Verification items for the finished model (mm, model axes). Give positions to 0.01 mm unless a question says otherwise; leave off trailing zeros. Write each loop counter-clockwise with the first axis right and the second up, starting at its lowest first coordinate (ties: lowest second). Pieces come first, ordered by that corner, then holes. Notation, with made-up numbers: (49, 38.5) -> (64, 38.5) arc R20 ccw to (64, 60.5) -> close; hole circle Ø1 at (-15.5, 3). An arc over 180 degrees is marked (long way). Use CSV: the item, a comma, the result in double quotes. Start each with the question number.
```python
from build123d import *

# Parameters (mm, degrees)
SKETCH_1_R              = 50
EXTRUDE_1_DEPTH         = 3.302
SKETCH_2_R              = 4.064
CUT_EXTRUDE_1_DEPTH     = 71.787733429
SKETCH_4_R              = 7.62
CUT_EXTRUDE_3_DEPTH     = 71.787733429
SKETCH_7_R              = 1.27
CUT_EXTRUDE_6_DEPTH     = 71.787733429
F_3_8_CLEARANCE_HOLE1_D = 10.0838
SKETCH11_R              = 1.9
CUT_EXTRUDE5_DEPTH      = 71.787733429
CIRPATTERN1_COUNT       = 2
SKETCH12_W              = 38.1
SKETCH12_H              = 9.525
CUT_EXTRUDE6_DEPTH      = 71.787733429
FILLET1_R               = 3.175
FILLET1_OF_MIRROR1_R    = 3.175


with BuildPart() as part:
    # 草图1 → 凸台-拉伸1 (new body)
    with BuildSketch(Plane.XY):
        with Locations(Location((0, 0, 0), (0, 0, 180))):
            Circle(SKETCH_1_R)
    extrude(amount=EXTRUDE_1_DEPTH)

    # 草图2 → 切除-拉伸1 (cut, through all)
    with BuildSketch(Plane.XY.offset(3.302)):
        with Locations((-26.940768363, 26.940768363)):
            Circle(SKETCH_2_R)
        with Locations((-26.940768363, -26.940768363)):
            Circle(SKETCH_2_R)
        with Locations((26.940768363, -26.940768363)):
            Circle(SKETCH_2_R)
        with Locations((26.940768363, 26.940768363)):
            Circle(SKETCH_2_R)
    extrude(amount=-CUT_EXTRUDE_1_DEPTH, mode=Mode.SUBTRACT)

    # 草图4 → 切除-拉伸3 (cut, through all)
    with BuildSketch(Plane.XY.offset(3.302)):
        Circle(SKETCH_4_R)
    extrude(amount=-CUT_EXTRUDE_3_DEPTH, mode=Mode.SUBTRACT)

    # 草图7 → 切除-拉伸6 (cut, through all)
    with BuildSketch(Plane.XY.offset(3.302)):
        with Locations((0, 46.99)):
            Circle(SKETCH_7_R)
        with Locations((46.99, 0)):
            Circle(SKETCH_7_R)
        with Locations((0, -46.99)):
            Circle(SKETCH_7_R)
        with Locations((-46.99, 0)):
            Circle(SKETCH_7_R)
    extrude(amount=-CUT_EXTRUDE_6_DEPTH, mode=Mode.SUBTRACT)

    # 3/8 Clearance Hole1 (through all)
    with Locations(Plane.XY.offset(3.302)):
        with Locations((0, 31.75), (-31.75, 0), (31.75, 0), (0, -31.75)):
            Hole(F_3_8_CLEARANCE_HOLE1_D / 2)

    # Sketch11 → Cut-Extrude5 (cut, through all)
    with BuildSketch(Plane.XY.offset(3.302)):
        with Locations((-16.51, 0)):
            Circle(SKETCH11_R)
    cut_extrude5 = extrude(amount=-CUT_EXTRUDE5_DEPTH, mode=Mode.SUBTRACT)

    # CirPattern1: Cut-Extrude5 ×2 about axis
    cirpattern1_axis = Axis((0, 0, 0), (0, 0, 1))
    for i in range(1, CIRPATTERN1_COUNT):
        add(cut_extrude5.rotate(cirpattern1_axis, i * 360 / CIRPATTERN1_COUNT), mode=Mode.SUBTRACT)

    # Sketch12 → Cut-Extrude6 (cut, through all)
    with BuildSketch(Plane.XY.offset(3.302)):
        with Locations((0, 17.145)):
            Rectangle(SKETCH12_W, SKETCH12_H)
    cut_extrude6 = extrude(amount=-CUT_EXTRUDE6_DEPTH, mode=Mode.SUBTRACT)

    # Fillet1
    fillet1_edges = [part.edges().sort_by_distance(p)[0] for p in [
        (19.05, 21.9075, 1.651),
        (19.05, 12.3825, 1.651),
        (-19.05, 12.3825, 1.651),
        (-19.05, 21.9075, 1.651),
    ]]
    fillet(fillet1_edges, radius=FILLET1_R)

    # Mirror1: Cut-Extrude6 across plane
    add(cut_extrude6.mirror(Plane.ZX), mode=Mode.SUBTRACT)

    # Fillet1 of Mirror1
    fillet1_of_mirror1_edges = [part.edges().sort_by_distance(p)[0] for p in [
        (19.05, -21.9075, 1.651),
        (19.05, -12.3825, 1.651),
        (-19.05, -12.3825, 1.651),
        (-19.05, -21.9075, 1.651),
    ]]
    fillet(fillet1_of_mirror1_edges, radius=FILLET1_OF_MIRROR1_R)


solid = part.part
```
(1) Section check C-C on z = 2.35. Give the number of separate pieces and of enclosed holes in the cut face, then the cut area to 3 significant figures.
(2) Section check D-D on x = 46.99. Record the cut outline in (y, z), then the cut area to 3 significant figures.
(3) Thickness scan on line 1 (X direction, y = -26, z = 1); line 2 (Y direction, x = -3.5, z = 3.25); line 3 (Y direction, x = 11, z = 0.1) (1 decimal). Record the ranges inside material, lowest first. Write a range as from..to.
(4) Section check B-B on y = -34.5. Record the cut outline in (x, z).
(5) Go/stop test with flat-tipped pins: pin 1 (20 mm diameter, centred on x = 0, y = 0, fed in from +Z); pin 2 (1.6 mm diameter, centred on y = 16.5, z = 2, fed in from +X); pin 3 (6 mm diameter, centred on x = -31.75, y = 0, fed in from -Z); pin 4 (1 mm diameter, centred on y = -21, z = 0.5, fed in from -X). Record where each tip stops, or that it passes through.
(6) Section check A-A on x = 29. Record the cut outline in (y, z), then the cut area to 3 significant figures.
Data:
1,separate pieces,"1"
1,enclosed holes,"17"
1,area,"6,390 mm2"
2,outline,"(-17.09, 0) -> (-1.27, 0) -> (-1.27, 3.3) -> (-17.09, 3.3) -> close; (1.27, 0) -> (17.09, 0) -> (17.09, 3.3) -> (1.27, 3.3) -> close"
2,area,"104 mm2"
3,line 1,"x = -42.71..-30.89, -22.99..22.99, 30.89..42.71"
3,line 2,"y = -49.88..-35.38, -28.12..-21.91, -12.38..-6.77, 6.77..12.38, 21.91..28.12, 35.38..49.88"
3,line 3,"y = -48.8..-21.9, -12.4..12.4, 21.9..48.8"
4,outline,"(-36.19, 0) -> (-4.23, 0) -> (-4.23, 3.3) -> (-36.19, 3.3) -> close; (4.23, 0) -> (36.19, 0) -> (36.19, 3.3) -> (4.23, 3.3) -> close"
5,pin 1,"stops at z = 3.3"
5,pin 2,"stops at x = 47.47"
5,pin 3,"passes through"
5,pin 4,"stops at x = -45.6"
6,outline,"(-40.73, 0) -> (-30.44, 0) -> (-30.44, 3.3) -> (-40.73, 3.3) -> close; (-23.44, 0) -> (-4.23, 0) -> (-4.23, 3.3) -> (-23.44, 3.3) -> close; (4.23, 0) -> (23.44, 0) -> (23.44, 3.3) -> (4.23, 3.3) -> close; (30.44, 0) -> (40.73, 0) -> (40.73, 3.3) -> (30.44, 3.3) -> close"
6,area,"195 mm2"
